```python
from build123d import *

# Parameters (mm, degrees)
SKETCH1_W               = 85
SKETCH1_H               = 56
BOSS_EXTRUDE1_DEPTH     = 3
SKETCH2_R               = 1.5
CUT_EXTRUDE1_DEPTH      = 1
CUT_EXTRUDE1_DEPTH_BACK = 4
FILLET1_R               = 3
SKETCH3_R               = 17.5
CUT_EXTRUDE2_DEPTH      = 1
CUT_EXTRUDE2_DEPTH_BACK = 4
SKETCH4_W               = 35
SKETCH4_H               = 20
BOSS_EXTRUDE2_DEPTH     = 3
FILLET2_R               = 5
CUT_EXTRUDE3_DEPTH      = 1
CUT_EXTRUDE3_DEPTH_BACK = 4


with BuildPart() as part:
    # Sketch1 → Boss-Extrude1 (new body)
    with BuildSketch(Plane(origin=(0, 0, 0), x_dir=(1, 0, 0), z_dir=(0, 1, 0))):
        Rectangle(SKETCH1_W, SKETCH1_H)
    extrude(amount=BOSS_EXTRUDE1_DEPTH)

    # Sketch2 → Cut-Extrude1 (cut, two sides)
    with BuildSketch(Plane(origin=(0, 3, 0), x_dir=(1, 0, 0), z_dir=(0, 1, 0))) as cut_extrude1_sk:
        with Locations((-39, 24.5)):
            Circle(SKETCH2_R)
        with Locations((19, 24.5)):
            Circle(SKETCH2_R)
        with Locations((19, -24.5)):
            Circle(SKETCH2_R)
        with Locations((-39, -24.5)):
            Circle(SKETCH2_R)
    extrude(amount=CUT_EXTRUDE1_DEPTH, mode=Mode.SUBTRACT)
    extrude(cut_extrude1_sk.sketch, amount=-CUT_EXTRUDE1_DEPTH_BACK, mode=Mode.SUBTRACT)

    # Fillet1
    fillet1_edges = [part.edges().sort_by_distance(p)[0] for p in [
        (42.5, 1.5, 28),
        (-42.5, 1.5, 28),
        (-42.5, 1.5, -28),
        (42.5, 1.5, -28),
    ]]
    fillet(fillet1_edges, radius=FILLET1_R)

    # Sketch3 → Cut-Extrude2 (cut, two sides)
    with BuildSketch(Plane(origin=(0, 3, 0), x_dir=(1, 0, 0), z_dir=(0, 1, 0))) as cut_extrude2_sk:
        with Locations((-10, 0)):
            Circle(SKETCH3_R)
    extrude(amount=CUT_EXTRUDE2_DEPTH, mode=Mode.SUBTRACT)
    extrude(cut_extrude2_sk.sketch, amount=-CUT_EXTRUDE2_DEPTH_BACK, mode=Mode.SUBTRACT)

    # Sketch4 → Boss-Extrude2 (add)
    with BuildSketch(Plane(origin=(0, 3, 0), x_dir=(1, 0, 0), z_dir=(0, 1, 0))):
        with Locations((0, 38)):
            Rectangle(SKETCH4_W, SKETCH4_H)
    extrude(amount=-BOSS_EXTRUDE2_DEPTH)

    # Fillet2
    fillet2_edges = [part.edges().sort_by_distance(p)[0] for p in [
        (17.5, 1.5, -48),
        (17.5, 1.5, -28),
        (-17.5, 1.5, -28),
        (-17.5, 1.5, -48),
    ]]
    fillet(fillet2_edges, radius=FILLET2_R)

    # Sketch5 → Cut-Extrude3 (cut, two sides)
    with BuildSketch(Plane(origin=(0, 3, 0), x_dir=(1, 0, 0), z_dir=(0, 1, 0))) as cut_extrude3_sk:
        with BuildLine():
            Line((-8, 40), (8, 40))
            ThreePointArc((8, 40), (10, 38), (8, 36))
            Line((8, 36), (-8, 36))
            ThreePointArc((-8, 36), (-10, 38), (-8, 40))
        make_face()
    extrude(amount=CUT_EXTRUDE3_DEPTH, mode=Mode.SUBTRACT)
    extrude(cut_extrude3_sk.sketch, amount=-CUT_EXTRUDE3_DEPTH_BACK, mode=Mode.SUBTRACT)


solid = part.part
```
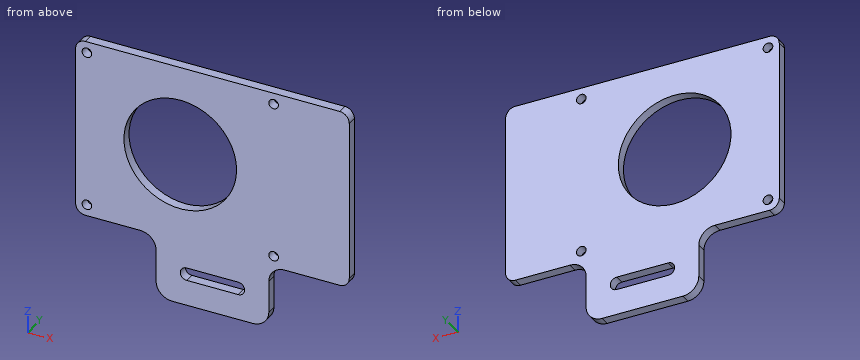
Could you check a few things on this model? Use its own coordinates, in mm. Round coordinates to 2 decimals unless told otherwise and drop trailing zeros. Order: outer loops, then holes, each group sorted by start corner. A loop starts at its lowest first (then second) coordinate and runs counter-clockwise, first axis right, second up. Notation, with made-up numbers: M -0.5,-5.75 L 22.5,-5.75 A10 ccw 22.5,7.25 Z; hole C -40,49 d5. An arc over 180 degrees is marked long. One line per question, with ' | ' between items. Start each with the question number.
(1) Suppose I cut it at B-B on z = -38. List the corners of the cut face in (x, y) for me.
(2) Suppose I cut it at C-C on z = 0. List the corners of the cut face in (x, y) for me, then the cut area to 3 significant figures.
(3) For P1, Ø4, axis at x = -39, z = 24.5, coming from the -Y side; P2, Ø1, axis at x = -24.5, z = -5, coming from the +Y side; P3, Ø0.9, axis at x = 29.5, y = 2, coming from the -Z side; P4, Ø1.5, axis at y = 1, z = -39, coming from the +X side, each with a flat end and sliding along its axis, tell me the tip position at first contact or that it passes through.
(4) Please list where these lines run through material, in increasing order: line 1 along Z through (x, y) = (-39, 1.1); line 2 along X through (y, z) = (1.8, -24.5); line 3 along Z through (x, y) = (6, 1).
(5) Suppose I cut it at A-A on y = 2.25. List the corners of the cut face in (x, z) for me, then the cut area to 3 significant figures.
Geometry results:
1) outline: M -17.5,0 L -10,0 L -10,3 L -17.5,3 Z; M 10,0 L 17.5,0 L 17.5,3 L 10,3 Z
2) outline: M -42.5,0 L -27.5,0 L -27.5,3 L -42.5,3 Z; M 7.5,0 L 42.5,0 L 42.5,3 L 7.5,3 Z | area: 150 mm²
3) P1: y = 0 | P2: through | P3: z = -28 | P4: x = 17.5
4) line 1: -28 to -26, -23 to 23, 26 to 28 | line 2: -42.5 to -40.5, -37.5 to 17.5, 20.5 to 42.5 | line 3: -48 to -40, -36 to -7.09, 7.09 to 28
5) outline: M -42.5,-25 A3 ccw -39.5,-28 L -22.5,-28 A5 cw -17.5,-33 L -17.5,-43 A5 ccw -12.5,-48 L 12.5,-48 A5 ccw 17.5,-43 L 17.5,-33 A5 cw 22.5,-28 L 39.5,-28 A3 ccw 42.5,-25 L 42.5,25 A3 ccw 39.5,28 L -39.5,28 A3 ccw -42.5,25 Z; hole C -39,-24.5 d3; hole C -39,24.5 d3; hole C -10,0 d35; hole M -8,-40 L 8,-40 A2 ccw 8,-36 L -8,-36 A2 ccw Z; hole C 19,-24.5 d3; hole C 19,24.5 d3 | area: 4,390 mm²
